```python
from build123d import *

# Parameters (mm, degrees)
F0_R     = 1.5
F1_DEPTH = 3


# Not quite as in the source:
# - a feature names something its author has since deleted; it is built from what else it names


with BuildPart() as f1:
    # F0 (on Front) → F1 (new body)
    with BuildSketch(Plane.XZ):
        with BuildLine():
            Line((7.5, 0), (11, 0))
            ThreePointArc((11, 0), (0, 11), (-11, 0))
            Line((-11, 0), (-7.5, 0))
            Line((-7.5, 0), (-7.5, -3))
            Line((-7.5, -3), (-4.5, -3))
            Line((-4.5, -3), (-4.5, 0))
            Line((-4.5, 0), (-1.5, 0))
            Line((-1.5, 0), (-1.5, -3))
            Line((-1.5, -3), (1.5, -3))
            Line((1.5, -3), (1.5, 0))
            Line((1.5, 0), (4.5, 0))
            Line((4.5, 0), (4.5, -3))
            Line((4.5, -3), (7.5, -3))
            Line((7.5, -3), (7.5, 0))
        make_face()
        with Locations((0, 5)):
            Circle(F0_R, mode=Mode.SUBTRACT)
    extrude(amount=F1_DEPTH)


solid = f1.part
```
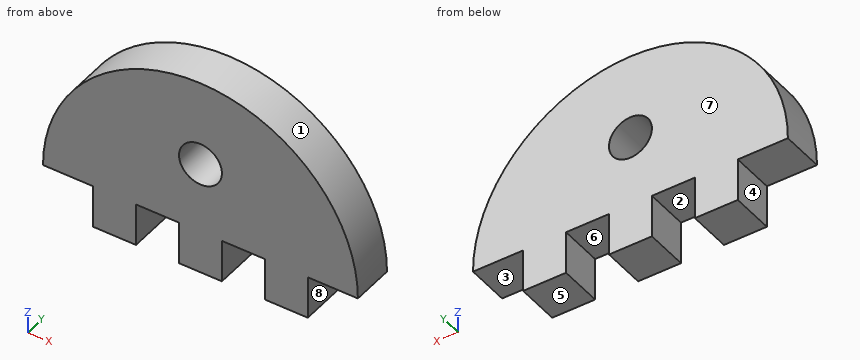
Can you work these out from the model? Positions are in its coordinate system, mm. Face numbers are marked on the shaded views. A direction names the side the tool comes from. Give positions to 0.01 mm unless a question says otherwise; leave off trailing zeros. Loops run counter-clockwise (first coordinate to the right, second up) from the corner with the lowest first, then second, coordinate; pieces in that order, holes last. Notation, with made-up numbers: M 29,6.5 L 83,6.5 A14 cw 83,11.5 Z; hole C 25,89 d9. An arc over 180 degrees is marked long. One line per question, with ' | ' between items. Start each with the question number.
Q1. If we section it at A-A (x = 0): Please give me the cut outline in (y, z).
Q2. If we section it at B-B (y = -1.1): Please give me the cut outline in (x, z), plus the area to 3 significant figures.
Q3. For pin 1 Ø1 at (x, y) = (-7, -1.5) entering from +Z; pin 2 Ø0.9 at (y, z) = (-1.5, -1.5) entering from +X; pin 3 Ø1.5 at (x, y) = (-3.5, -1.5) entering from -Z, each with a flat end and sliding along its axis, tell me the tip position at first contact or that it passes through.
Q4. If we section it at D-D (z = 5): Please give me the cut outline in (x, y), plus the area to 3 significant figures.
Q5. For the marked faces 1, 2, 3, 4 and 5, which set-ups out of +Z, -Z, +X, -X, +Y, -Y let a thin tool reach every point of the face, with its end or its side?
Q6. If I drill on line 1 (X direction, y = -1.85, z = -1.25); line 2 (Z direction, x = 0, y = -2); line 3 (X direction, y = -0.15, z = 5.5), over which ranges is the centre line in solid material (lowest first)? Write a range as from..to.
Q7. If we section it at C-C (z = -1.25): Please give me the cut outline in (x, y).
Q8. If we mould it in two halves opening along X, with no side actions, what happens to the marked faces 6, 7 and 8? For each: +X half, -X half, draft (parallel to the pull), parting line (faces both ways), or undercut.
Computed:
1) outline: M -3,-3 L 0,-3 L 0,3.5 L -3,3.5 Z; M -3,6.5 L 0,6.5 L 0,11 L -3,11 Z
2) outline: M -11,0 L -7.5,0 L -7.5,-3 L -4.5,-3 L -4.5,0 L -1.5,0 L -1.5,-3 L 1.5,-3 L 1.5,0 L 4.5,0 L 4.5,-3 L 7.5,-3 L 7.5,0 L 11,0 A11 ccw Z; hole C 0,5 d3 | area: 210 mm²
3) pin 1: stops at z = 8.87 | pin 2: stops at x = 7.5 | pin 3: stops at z = 0
4) outline: M -9.8,-3 L -1.5,-3 L -1.5,0 L -9.8,0 Z; M 1.5,-3 L 9.8,-3 L 9.8,0 L 1.5,0 Z | area: 49.8 mm²
5) face 1: +Z, +Y, -Y | face 2: -Z, +Y, -Y | face 3: -Z, +X, +Y, -Y | face 4: -Z, -X, +Y, -Y | face 5: -Z, +X, -X, +Y, -Y
6) line 1: x = -7.5..-4.5, -1.5..1.5, 4.5..7.5 | line 2: z = -3..3.5, 6.5..11 | line 3: x = -9.53..-1.41, 1.41..9.53
7) outline: M -7.5,-3 L -4.5,-3 L -4.5,0 L -7.5,0 Z; M -1.5,-3 L 1.5,-3 L 1.5,0 L -1.5,0 Z; M 4.5,-3 L 7.5,-3 L 7.5,0 L 4.5,0 Z
8) face 6: undercut | face 7: draft | face 8: +X half
